from build123d import *

# Parameters (mm, degrees)
SKETCH1_W                = 32
SKETCH1_H                = 29
BOSS_EXTRUDE1_DEPTH      = 35
FILLET1_R                = 2
SLOT_FOR_COIL_DEPTH      = 1
SLOT_FOR_COIL_DEPTH_BACK = 30
BOSS_EXTRUDE2_DEPTH      = 7
BOSS_EXTRUDE3_DEPTH      = 1.75
SKETCH5_W                = 2
SKETCH5_H                = 7
CUT_EXTRUDE2_DEPTH       = 33
CUT_EXTRUDE3_DEPTH       = 22
SKETCH7_W                = 2
SKETCH7_H                = 33
BOSS_EXTRUDE4_DEPTH      = 0.25
FILLET2_R                = 6
CUT_EXTRUDE5_DEPTH       = 4.5
SKETCH14_W               = 2.5
SKETCH14_H               = 20
CUT_EXTRUDE6_DEPTH       = 22
SKETCH16_W               = 2
SKETCH16_H               = 2
BOSS_EXTRUDE5_DEPTH      = 22
BOSS_EXTRUDE6_DEPTH      = 22
SKETCH21_W               = 10
SKETCH21_H               = 2
BOSS_EXTRUDE7_DEPTH      = 3
SKETCH23_W               = 8
SKETCH23_H               = 1.75
CUT_EXTRUDE7_DEPTH       = 2
FILLET3_R                = 1
CUT_EXTRUDE8_REACH       = 34
SKETCH26_R               = 5


with BuildPart() as part:
    # Sketch1 → Boss-Extrude1 (new body)
    with BuildSketch(Plane.XY):
        Rectangle(SKETCH1_W, SKETCH1_H)
    extrude(amount=BOSS_EXTRUDE1_DEPTH)

    # Fillet1
    fillet1_edges = [part.edges().sort_by_distance(p)[0] for p in [
        (16, -14.5, 17.5),
        (-16, -14.5, 17.5),
        (-16, 14.5, 17.5),
        (16, 14.5, 17.5),
    ]]
    fillet(fillet1_edges, radius=FILLET1_R)

    # Sketch2 → Slot for Coil (cut, two sides)
    with BuildSketch(Plane.XZ.offset(14.5)) as slot_for_coil_sk:
        Polygon((-9.125, 0), (-9.125, 1.75), (-11.125, 1.75), (-11.125, 5), (11.125, 5), (11.125, 1.75), (9.125, 1.75), (9.125, 0), align=None)
    extrude(amount=SLOT_FOR_COIL_DEPTH, mode=Mode.SUBTRACT)
    extrude(slot_for_coil_sk.sketch, amount=-SLOT_FOR_COIL_DEPTH_BACK, mode=Mode.SUBTRACT)

    # Sketch3 → Boss-Extrude2 (add)
    with BuildSketch(Plane.XZ.offset(14.5)):
        Polygon((-9.125, 0), (-9.125, 1.75), (-11.125, 1.75), (-11.125, 5), (11.125, 5), (11.125, 1.75), (9.125, 1.75), (9.125, 0), align=None)
    extrude(amount=-BOSS_EXTRUDE2_DEPTH)

    # Sketch4 → Boss-Extrude3 (add)
    with BuildSketch(Plane(origin=(0, 0, 1.75), x_dir=(-1, 0, 0), z_dir=(0, 0, -1))):
        with BuildLine():
            Line((-9.125, 7.5), (-9.125, 6.5))
            ThreePointArc((-9.125, 6.5), (-8.875, 7), (-9.125, 7.5))
        make_face()
    boss_extrude3 = extrude(amount=BOSS_EXTRUDE3_DEPTH)

    # Mirror1: Boss-Extrude3 across plane
    add(boss_extrude3.mirror(Plane(origin=(0, 0, 0), x_dir=(0, 0, 1), z_dir=(1, 0, 0))))

    # Sketch5 → Cut-Extrude2 (cut)
    with BuildSketch(Plane(origin=(0, 0, 0), x_dir=(-1, 0, 0), z_dir=(0, 0, -1))):
        with Locations((0, -11)):
            Rectangle(SKETCH5_W, SKETCH5_H)
    extrude(amount=-CUT_EXTRUDE2_DEPTH, mode=Mode.SUBTRACT)

    # Sketch6 → Cut-Extrude3 (cut)
    with BuildSketch(Plane(origin=(0, 14.5, 0), x_dir=(1, 0, 0), z_dir=(0, 1, 0))):
        Polygon((-12.5, -7.5), (-12.5, -11), (-11.5, -11), (-11.5, -33), (11.5, -33), (11.5, -11), (12.5, -11), (12.5, -7.5), align=None)
    extrude(amount=-CUT_EXTRUDE3_DEPTH, mode=Mode.SUBTRACT)

    # Sketch7 → Boss-Extrude4 (add)
    with BuildSketch(Plane.XZ.offset(14.5)):
        with Locations((0, 16.5)):
            Rectangle(SKETCH7_W, SKETCH7_H)
    extrude(amount=-BOSS_EXTRUDE4_DEPTH)

    # Fillet2
    fillet2_edges = [part.edges().sort_by_distance(p)[0] for p in [
        (0, -14.25, 33),
    ]]
    fillet(fillet2_edges, radius=FILLET2_R)

    # Sketch11 → Cut-Extrude5 (cut)
    with BuildSketch(Plane(origin=(-16, 0, 44), x_dir=(0, 0, -1), z_dir=(1, 0, 0))):
        with BuildLine():
            Line((27, 25), (27, 0))
            ThreePointArc((27, 0), (21, -6), (15, 0))
            Line((15, 0), (15, 25))
            ThreePointArc((15, 25), (21, 31), (27, 25))
        make_face()
    extrude(amount=CUT_EXTRUDE5_DEPTH, mode=Mode.SUBTRACT)

    # Sketch14 → Cut-Extrude6 (cut)
    with BuildSketch(Plane(origin=(0, 14.5, 0), x_dir=(1, 0, 0), z_dir=(0, 1, 0))):
        with Locations((-12.75, -23)):
            Rectangle(SKETCH14_W, SKETCH14_H)
    extrude(amount=-CUT_EXTRUDE6_DEPTH, mode=Mode.SUBTRACT)

    # Sketch16 → Boss-Extrude5 (add)
    with BuildSketch(Plane(origin=(0, 14.5, 0), x_dir=(1, 0, 0), z_dir=(0, 1, 0))):
        with Locations((-11, -14)):
            Rectangle(SKETCH16_W, SKETCH16_H)
        with Locations((-11, -32)):
            Rectangle(SKETCH16_W, SKETCH16_H)
    extrude(amount=-BOSS_EXTRUDE5_DEPTH)

    # Sketch20 → Boss-Extrude6 (add)
    with BuildSketch(Plane(origin=(0, 14.5, 0), x_dir=(1, 0, 0), z_dir=(0, 1, 0))):
        Polygon((-11.5, -11), (-10, -13), (-11.5, -13), align=None)
        Polygon((-10, -31), (-8.5, -33), (-10, -33), align=None)
    extrude(amount=-BOSS_EXTRUDE6_DEPTH)

    # Sketch21 → Boss-Extrude7 (add)
    with BuildSketch(Plane(origin=(0, 14.5, 0), x_dir=(-1, 0, 0), z_dir=(0, 1, 0))):
        with Locations((0, 34)):
            Rectangle(SKETCH21_W, SKETCH21_H)
    boss_extrude7 = extrude(amount=BOSS_EXTRUDE7_DEPTH)

    # Sketch23 → Cut-Extrude7 (cut)
    with BuildSketch(Plane.XY.offset(35)):
        with Locations((0, 16.125)):
            Rectangle(SKETCH23_W, SKETCH23_H)
    cut_extrude7 = extrude(amount=-CUT_EXTRUDE7_DEPTH, mode=Mode.SUBTRACT)

    # Mirror3: Boss-Extrude7, Cut-Extrude7 across plane
    add(boss_extrude7.mirror(Plane.ZX))
    add(cut_extrude7.mirror(Plane.ZX), mode=Mode.SUBTRACT)

    # Fillet3
    fillet3_edges = [part.edges().sort_by_distance(p)[0] for p in [
        (5, 14.5, 34),
        (-5, 14.5, 34),
        (5, 17.5, 34),
        (-5, 17.5, 34),
        (5, -17.5, 34),
        (-5, -17.5, 34),
        (5, -14.5, 34),
        (-5, -14.5, 34),
    ]]
    fillet(fillet3_edges, radius=FILLET3_R)

    # Sketch26 → Cut-Extrude8 (cut, up to next)
    with BuildSketch(Plane(origin=(16, 0, 0), x_dir=(0, 0, -1), z_dir=(1, 0, 0)), mode=Mode.PRIVATE) as cut_extrude8_sk1:
        with Locations((-17.485, -2.89)):
            Circle(SKETCH26_R)
    cut_extrude8_tool1 = extrude(cut_extrude8_sk1.sketch, amount=-CUT_EXTRUDE8_REACH, mode=Mode.PRIVATE) & part.part
    add(cut_extrude8_tool1.solids().sort_by_distance((16, -2.89, 17.485))[0], mode=Mode.SUBTRACT)


solid = part.part
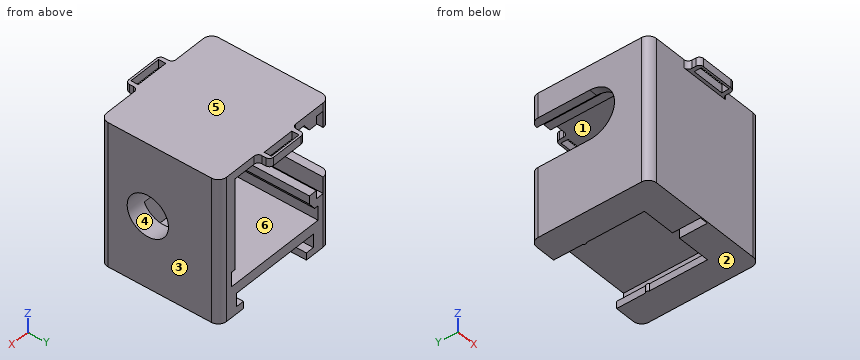
Geometry check sheet. Reference: the model listing, model coordinates, mm. Face numbers are marked on the shaded views. A direction names the side the tool comes from. Round coordinates to 2 decimals unless told otherwise and drop trailing zeros. Loops run counter-clockwise (first coordinate to the right, second up) from the corner with the lowest first, then second, coordinate; pieces in that order, holes last. Notation, with made-up numbers: (-37, 65.25) -> (-1, 65.25) arc R22 cw to (-1, 85.25) -> close; hole circle Ø1 at (44.25, 4). An arc over 180 degrees is marked (long way). Answer as a JSON object with one key per item and string values. Group by question number.
Item 1: Release check for a two-part mould opening along X. For the marked faces 1, 2 and 3 record: pulls with the +X half, pulls with the -X half, needs draft (parallel to the pull), parting line crosses it, or undercut.
Item 2: Thickness scan on line 1 along Z through (x, y) = (11, -2.89); line 2 along Z through (x, y) = (-8, -6); line 3 along X through (y, z) = (-2.5, 2) (3 decimals). Record the ranges inside material, lowest first.
Item 3: Cross-section at A-A, the plane x = 2. Record the cut outline in (y, z) (3 decimals).
Item 4: Cross-section at C-C, the plane x = -2. Record the cut outline in (y, z), plus the area to 3 significant figures.
Item 5: Set-up check for the marked faces 4, 5 and 6: record each of +Z, -Z, +X, -X, +Y, -Y from which the full face is reachable in a straight line by a thin tool's end or side.
Item 6: Cross-section at B-B, the plane z = 23. Record the cut outline in (x, y), plus the area to 3 significant figures.
Item 7: Depth check by flat-ended pin: pin 1 Ø12 at (x, z) = (3, 9) entering from +Y; pin 2 Ø12 at (x, z) = (-4, 23) entering from +Y; pin 3 Ø1.4 at (y, z) = (-16, 33.5) entering from -X. Enter the tip coordinate at first touch or a pass-through.
Determined:
{
 "1": {"face 1": "undercut", "face 2": "needs draft", "face 3": "pulls with the +X half"},
 "2": {"line 1": "z = 0 to 1.75, 5 to 7.5, 33 to 35", "line 2": "z = 5 to 7.5, 33 to 35", "line 3": "x = -16 to -11.125, 11.125 to 16"},
 "3": {"outline": "(-17.5, 33) -> (-17, 33) -> (-17, 35) -> (-17.5, 35) -> close; (-15.25, 33) -> (-14.5, 33) -> (-14.5, 0) -> (-7.5, 0) -> (-7.5, 5) -> (14.5, 5) -> (14.5, 7.5) -> (-7.5, 7.5) -> (-7.5, 15.549) arc R5 cw to (-7.5, 19.421) -> (-7.5, 33) -> (15.25, 33) -> (15.25, 35) -> (-15.25, 35) -> close; (17, 33) -> (17.5, 33) -> (17.5, 35) -> (17, 35) -> close"},
 "4": {"outline": "(-17.5, 33) -> (-17, 33) -> (-17, 35) -> (-17.5, 35) -> close; (-15.25, 33) -> (-14.5, 33) -> (-14.5, 0) -> (-7.5, 0) -> (-7.5, 5) -> (14.5, 5) -> (14.5, 7.5) -> (-7.5, 7.5) -> (-7.5, 33) -> (15.25, 33) -> (15.25, 35) -> (-15.25, 35) -> close; (17, 33) -> (17.5, 33) -> (17.5, 35) -> (17, 35) -> close", "area": "349 mm²"},
 "5": {"face 4": "+X", "face 5": "+Z, +X, -X, +Y, -Y", "face 6": "+Y"},
 "6": {"outline": "(-16, -12.5) arc R2 ccw to (-14, -14.5) -> (14, -14.5) arc R2 ccw to (16, -12.5) -> (16, 12.5) arc R2 ccw to (14, 14.5) -> (11.5, 14.5) -> (11.5, -7.5) -> (1, -7.5) -> (1, -14.25) -> (-1, -14.25) -> (-1, -7.5) -> (-14, -7.5) -> (-14, -6) -> (-16, -6) -> close", "area": "310 mm²"},
 "7": {"pin 1": "stops at y = 14.5", "pin 2": "stops at y = -7.5", "pin 3": "stops at x = -5.02"}
}
